from build123d import *

# Parameters (mm, degrees)
BOSS_EXTRUDE1_DEPTH = 76.2
SKETCH2_R           = 6.35
CUT_EXTRUDE1_DEPTH  = 111.449174947
FILLET1_R           = 2.54


with BuildPart() as part:
    # Sketch1 → Boss-Extrude1 (new body)
    with BuildSketch(Plane.XY):
        Polygon((-56.707964559, -12.7), (70.292035441, -12.7), (70.292035441, 25.4), (25.842035441, 25.4), (25.842035441, 0), (-12.257964559, 0), (-12.257964559, 25.4), (-56.707964559, 25.4), align=None)
    extrude(amount=BOSS_EXTRUDE1_DEPTH)

    # Sketch2 → Cut-Extrude1 (cut, through all)
    with BuildSketch(Plane(origin=(0, 25.4, 0), x_dir=(1, 0, 0), z_dir=(0, 1, 0))):
        with Locations(Location((-37.657964559, -19.05, 0), (0, 0, 180))):
            Circle(SKETCH2_R)
        with Locations(Location((-37.657964559, -57.15, 0), (0, 0, 180))):
            Circle(SKETCH2_R)
        with Locations(Location((51.242035441, -19.05, 0), (0, 0, 180))):
            Circle(SKETCH2_R)
        with Locations(Location((51.242035441, -57.15, 0), (0, 0, 180))):
            Circle(SKETCH2_R)
    extrude(amount=-CUT_EXTRUDE1_DEPTH, mode=Mode.SUBTRACT)

    # Fillet1
    fillet1_edges = [part.edges().sort_by_distance(p)[0] for p in [
        (-34.482964559, 25.4, 0),
        (-12.257964559, 25.4, 38.1),
        (25.842035441, 25.4, 38.1),
        (70.292035441, 25.4, 38.1),
        (-56.707964559, 25.4, 38.1),
        (48.067035441, 25.4, 76.2),
        (-31.307964559, 25.4, 57.15),
        (57.592035441, 25.4, 19.05),
        (57.592035441, 25.4, 57.15),
        (-31.307964559, 25.4, 19.05),
        (-34.482964559, 25.4, 76.2),
        (48.067035441, 25.4, 0),
    ]]
    fillet(fillet1_edges, radius=FILLET1_R)


solid = part.part
The model under review builds one solid part; all positions refer to its coordinate system, in mm. A direction names the side the tool comes from. Round coordinates to 2 decimals unless told otherwise and drop trailing zeros. Loops run counter-clockwise (first coordinate to the right, second up) from the corner with the lowest first, then second, coordinate; pieces in that order, holes last. Notation, with made-up numbers: (18, 82.5) -> (46, 82.5) arc R15 cw to (46, 108.5) -> close; hole circle Ø9 at (68.5, 88). An arc over 180 degrees is marked (long way). Return JSON: item names as keys, results as strings.
(1) Add section D-D on x = 23. Write out the cut boundary in (y, z).
Solved:
{"outline": "(-12.7, 0) -> (0, 0) -> (0, 76.2) -> (-12.7, 76.2) -> close"}
(2) The part is to be moulded in two halves that separate along Z. For faces 1 (the cylindrical face through (47.756, 24.636, 0.724)), 2 (the flat face through (-56.708, 5, 38)), 3 (the cylindrical face through (-31.314, 5.329, 19.329)), say which applies: released by +Z, released by -Z, zero draft, split by the parting line, or undercut.
Solved:
{"face 1": "released by -Z", "face 2": "zero draft", "face 3": "undercut"}
(3) For faces 4 (the flat face through (6, -12.7, 38)), 5 (the flat face through (-12.258, 11, 38)), list the 3-axis set-ups (+Z, -Z, +X, -X, +Y, -Y) from which the entire face can be reached by the end or side of a thin tool; tool diameter is ignored.
Solved:
{"face 4": "+Z, -Z, +X, -X, -Y", "face 5": "+Z, -Z, +Y"}
(4) For line 1 (X direction, y = 6, z = 19); line 2 (Z direction, x = 47.5, y = 23.5); line 3 (X direction, y = -11, z = 16), list the stretches that pass through material, from the lowest coordinate up.
Solved:
{"line 1": "-56.71 to -44.01, -31.31 to -12.26, 25.84 to 44.89, 57.59 to 70.29", "line 2": "0.08 to 13.82, 24.28 to 51.92, 62.38 to 76.12", "line 3": "-56.71 to -43.23, -32.09 to 45.67, 56.81 to 70.29"}
(5) Add section A-A on y = 5.5. Write out the cut boundary in (x, z), plus the area to 3 significant figures.
Solved:
{"outline": "(-56.71, 0) -> (-12.26, 0) -> (-12.26, 76.2) -> (-56.71, 76.2) -> close; (25.84, 0) -> (70.29, 0) -> (70.29, 76.2) -> (25.84, 76.2) -> close; hole circle Ø12.7 at (-37.66, 19.05); hole circle Ø12.7 at (-37.66, 57.15); hole circle Ø12.7 at (51.24, 19.05); hole circle Ø12.7 at (51.24, 57.15)", "area": "6,270 mm2"}
(6) For pin 1 (16.5 mm diameter, centred on x = 51.24, z = 19.05, fed in from +Y); pin 2 (16.5 mm diameter, centred on x = -37.66, z = 19.05, fed in from -Y), all flat-tipped, find the tip position at first contact; note any pin that passes through.
Solved:
{"pin 1": "y = 25.32", "pin 2": "y = -12.7"}
(7) Add section B-B on z = 19.05. Write out the cut boundary in (x, y), plus the area to 3 significant figures.
Solved:
{"outline": "(-56.71, -12.7) -> (-44.01, -12.7) -> (-44.01, 22.86) arc R2.54 ccw to (-46.55, 25.4) -> (-54.17, 25.4) arc R2.54 ccw to (-56.71, 22.86) -> close; (-31.31, -12.7) -> (44.89, -12.7) -> (44.89, 22.86) arc R2.54 ccw to (42.35, 25.4) -> (28.38, 25.4) arc R2.54 ccw to (25.84, 22.86) -> (25.84, 0) -> (-12.26, 0) -> (-12.26, 22.86) arc R2.54 ccw to (-14.8, 25.4) -> (-28.77, 25.4) arc R2.54 ccw to (-31.31, 22.86) -> close; (57.59, -12.7) -> (70.29, -12.7) -> (70.29, 22.86) arc R2.54 ccw to (67.75, 25.4) -> (60.13, 25.4) arc R2.54 ccw to (57.59, 22.86) -> close", "area": "2,890 mm2"}
(8) Add section C-C on y = -5.5. Write out the cut boundary in (x, z).
Solved:
{"outline": "(-56.71, 0) -> (70.29, 0) -> (70.29, 76.2) -> (-56.71, 76.2) -> close; hole circle Ø12.7 at (-37.66, 19.05); hole circle Ø12.7 at (-37.66, 57.15); hole circle Ø12.7 at (51.24, 19.05); hole circle Ø12.7 at (51.24, 57.15)"}
